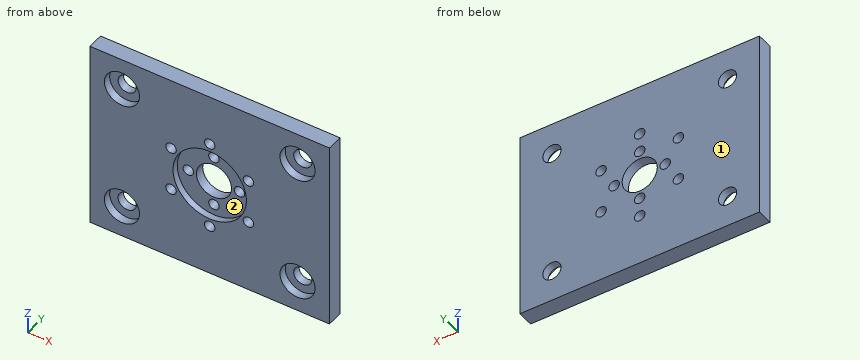
from build123d import *

# Parameters (mm, degrees)
SKETCH_1_W               = 75
SKETCH_1_H               = 60
EXTRUDE_1_DEPTH          = 5
HOLE_WIZARD_1_D          = 5.7
CUT_EXTRUDE_1_DEPTH      = 10
HOLE_WIZARD_2_D          = 3.3
PATTERN_CIRCULAR_1_COUNT = 6
HOLE_WIZARD_3_D          = 11
HOLE_WIZARD_3_DEPTH      = 2.5
HOLE_WIZARD_4_D          = 3.3
HOLE_WIZARD_5_D          = 23
HOLE_WIZARD_5_DEPTH      = 2


with BuildPart() as part:
    # 草图1 → 凸台-拉伸1 (new body)
    with BuildSketch(Plane(origin=(0, 0, 0), x_dir=(1, 0, 0), z_dir=(0, 1, 0))):
        with Locations((37.5, 30)):
            Rectangle(SKETCH_1_W, SKETCH_1_H)
    extrude(amount=EXTRUDE_1_DEPTH)

    # 孔1 (through all)
    with Locations(Plane(origin=(0, 5, 0), x_dir=(1, 0, 0), z_dir=(0, 1, 0))):
        with Locations((10, 50), (10, 10), (65, 10), (65, 50)):
            Hole(HOLE_WIZARD_1_D / 2)

    # 草图6 → 切除-拉伸1 (cut)
    with BuildSketch(Plane(origin=(0, 5, 0), x_dir=(1, 0, 0), z_dir=(0, 1, 0))):
        with BuildLine():
            ThreePointArc((43, 30), (37.5, 35.5), (32, 30))
            Line((32, 30), (43, 30))
        make_face()
        with BuildLine():
            Line((43, 30), (32, 30))
            ThreePointArc((32, 30), (37.5, 24.5), (43, 30))
        make_face()
    extrude(amount=-CUT_EXTRUDE_1_DEPTH, mode=Mode.SUBTRACT)

    # 孔2 (through all)
    with Locations(Plane(origin=(0, 5, 0), x_dir=(1, 0, 0), z_dir=(0, 1, 0))):
        with Locations((37.5, 44)):
            hole_wizard_2 = Hole(HOLE_WIZARD_2_D / 2)

    # 阵列(圆周)1: 孔2 ×6 about axis
    pattern_circular_1_axis = Axis((37.5, 0, -30), (0, 1, 0))
    for i in range(1, PATTERN_CIRCULAR_1_COUNT):
        add(hole_wizard_2.rotate(pattern_circular_1_axis, i * 360 / PATTERN_CIRCULAR_1_COUNT), mode=Mode.SUBTRACT)

    # 孔3
    with Locations(Plane(origin=(0, 0, 0), x_dir=(-1, 0, 0), z_dir=(0, -1, 0))):
        with Locations((-10, 10), (-10, 50), (-65, 50), (-65, 10)):
            Hole(HOLE_WIZARD_3_D / 2, depth=HOLE_WIZARD_3_DEPTH)

    # 孔4 (through all)
    with Locations(Plane(origin=(0, 5, 0), x_dir=(1, 0, 0), z_dir=(0, 1, 0))):
        with Locations((29.5, 30), (37.5, 38), (45.5, 30), (37.5, 22)):
            Hole(HOLE_WIZARD_4_D / 2)

    # 孔5
    with Locations(Plane(origin=(0, 0, 0), x_dir=(-1, 0, 0), z_dir=(0, -1, 0))):
        with Locations((-37.5, 30)):
            Hole(HOLE_WIZARD_5_D / 2, depth=HOLE_WIZARD_5_DEPTH)


solid = part.part
Verification items for the finished model (mm, model axes). Face numbers are marked on the shaded views. Coordinates: 2 decimals unless noted, no trailing zeros. Order: outer loops, then holes, each group sorted by start corner. A loop starts at its lowest first (then second) coordinate and runs counter-clockwise, first axis right, second up. Notation, with made-up numbers: (77, 24.25) -> (131, 24.25) arc R20 ccw to (131, 36.25) -> close; hole circle Ø2 at (34.25, -2). An arc over 180 degrees is marked (long way). Use CSV: the item, a comma, the result in double quotes. Start each with the question number.
Q1. Draft check along Z on the marked faces 1 and 2. Enter one of: +Z half, -Z half, draft (parallel to the pull), parting line (faces both ways), or undercut.
Q2. Depth check by flat-ended pin: P1, Ø5.5, axis at x = 67, z = -51.5, coming from the -Y side. Enter the tip coordinate at first touch or a pass-through.
Q3. Section check A-A, the plane x = 65. Record the cut outline in (y, z).
Q4. Section check C-C, the plane x = 37.5. Record the cut outline in (y, z), and give its area (3 significant figures).
Q5. Section check D-D, the plane z = -34. Record the cut outline in (x, y).
Q6. Section check B-B, the plane z = -50. Record the cut outline in (x, y).
Q7. Thickness scan on line 1 along Z through (x, y) = (10, 1.3); line 2 along X through (y, z) = (4.4, -10); line 3 along X through (y, z) = (1.7, -50). Record the ranges inside material, lowest first.
Returned:
1,face 1,"draft"
1,face 2,"undercut"
2,P1,"stops at y = 2.5"
3,outline,"(0, -60) -> (5, -60) -> (5, -52.85) -> (2.5, -52.85) -> (2.5, -55.5) -> (0, -55.5) -> close; (0, -44.5) -> (2.5, -44.5) -> (2.5, -47.15) -> (5, -47.15) -> (5, -12.85) -> (2.5, -12.85) -> (2.5, -15.5) -> (0, -15.5) -> close; (0, -4.5) -> (2.5, -4.5) -> (2.5, -7.15) -> (5, -7.15) -> (5, 0) -> (0, 0) -> close"
4,outline,"(0, -60) -> (5, -60) -> (5, -45.65) -> (0, -45.65) -> close; (0, -42.35) -> (5, -42.35) -> (5, -39.65) -> (2, -39.65) -> (2, -41.5) -> (0, -41.5) -> close; (0, -18.5) -> (2, -18.5) -> (2, -20.35) -> (5, -20.35) -> (5, -17.65) -> (0, -17.65) -> close; (0, -14.35) -> (5, -14.35) -> (5, 0) -> (0, 0) -> close; (2, -36.35) -> (5, -36.35) -> (5, -35.5) -> (2, -35.5) -> close; (2, -24.5) -> (5, -24.5) -> (5, -23.65) -> (2, -23.65) -> close"
4,area,"168 mm^2"
5,outline,"(0, 0) -> (26.72, 0) -> (26.72, 2) -> (33.73, 2) -> (33.73, 5) -> (0, 5) -> close; (41.27, 2) -> (48.28, 2) -> (48.28, 0) -> (75, 0) -> (75, 5) -> (41.27, 5) -> close"
6,outline,"(0, 0) -> (4.5, 0) -> (4.5, 2.5) -> (7.15, 2.5) -> (7.15, 5) -> (0, 5) -> close; (12.85, 2.5) -> (15.5, 2.5) -> (15.5, 0) -> (59.5, 0) -> (59.5, 2.5) -> (62.15, 2.5) -> (62.15, 5) -> (12.85, 5) -> close; (67.85, 2.5) -> (70.5, 2.5) -> (70.5, 0) -> (75, 0) -> (75, 5) -> (67.85, 5) -> close"
7,line 1,"z = -60 to -55.5, -44.5 to -15.5, -4.5 to 0"
7,line 2,"x = 0 to 7.15, 12.85 to 62.15, 67.85 to 75"
7,line 3,"x = 0 to 4.5, 15.5 to 59.5, 70.5 to 75"
